Geometry: final body of the model. Coordinates: model frame, mm. A direction names the side the tool comes from. Give positions to 0.01 mm unless a question says otherwise; leave off trailing zeros. Write each loop counter-clockwise with the first axis right and the second up, starting at its lowest first coordinate (ties: lowest second). Pieces come first, ordered by that corner, then holes. Notation, with made-up numbers: M 74.25,-19 L 90.25,-19 A12 cw 90.25,-10 Z; hole C 31,58.25 d9. An arc over 180 degrees is marked long. One line per question, with ' | ' between items.
from build123d import *

# Parameters (mm, degrees)
SKETCH1_W           = 40
SKETCH1_H           = 20
BOSS_EXTRUDE1_DEPTH = 37
BOSS_EXTRUDE2_DEPTH = 2
SKETCH3_W           = 3
SKETCH3_H           = 20
BOSS_EXTRUDE3_DEPTH = 7
SKETCH4_W           = 3
SKETCH4_H           = 20
BOSS_EXTRUDE4_DEPTH = 7
SKETCH8_R           = 2.15
CUT_EXTRUDE9_DEPTH  = 7
CUT_EXTRUDE10_REACH = 44.308
SKETCH9_R           = 2.15
CUT_EXTRUDE11_REACH = 44.308
SKETCH10_R          = 2.15
SKETCH11_R          = 3
BOSS_EXTRUDE5_DEPTH = 6


with BuildPart() as part:
    # Sketch1 → Boss-Extrude1 (new body)
    with BuildSketch(Plane.XY):
        Rectangle(SKETCH1_W, SKETCH1_H)
    extrude(amount=BOSS_EXTRUDE1_DEPTH)

    # Sketch2 → Boss-Extrude2 (add)
    with BuildSketch(Plane.XY.offset(37)):
        with BuildLine():
            Line((15, 10), (15, -10))
            Line((15, -10), (-10, -10))
            ThreePointArc((-10, -10), (-20, 0), (-10, 10))
            Line((-10, 10), (15, 10))
        make_face()
    extrude(amount=BOSS_EXTRUDE2_DEPTH)

    # Sketch3 → Boss-Extrude3 (add)
    with BuildSketch(Plane(origin=(20, 0, 0), x_dir=(0, 0, -1), z_dir=(1, 0, 0))):
        with Locations((-29.5, 0)):
            Rectangle(SKETCH3_W, SKETCH3_H)
    extrude(amount=BOSS_EXTRUDE3_DEPTH)

    # Sketch4 → Boss-Extrude4 (add)
    with BuildSketch(Plane.ZY.offset(20)):
        with Locations((29.5, 0)):
            Rectangle(SKETCH4_W, SKETCH4_H)
    extrude(amount=BOSS_EXTRUDE4_DEPTH)

    # Sketch8 → Cut-Extrude9 (cut)
    with BuildSketch(Plane.XY.offset(31)):
        with Locations((-25, 6)):
            Circle(SKETCH8_R)
    extrude(amount=-CUT_EXTRUDE9_DEPTH, mode=Mode.SUBTRACT)

    # Sketch9 → Cut-Extrude10 (cut, up to next)
    with BuildSketch(Plane.XY.offset(31), mode=Mode.PRIVATE) as cut_extrude10_sk1:
        with Locations((-25, -6)):
            Circle(SKETCH9_R)
    cut_extrude10_tool1 = extrude(cut_extrude10_sk1.sketch, amount=-CUT_EXTRUDE10_REACH, mode=Mode.PRIVATE) & part.part
    add(cut_extrude10_tool1.solids().sort_by_distance((-25, -6, 31))[0], mode=Mode.SUBTRACT)

    # Sketch10 → Cut-Extrude11 (cut, up to next)
    with BuildSketch(Plane.XY.offset(31), mode=Mode.PRIVATE) as cut_extrude11_sk1:
        with Locations((25, 6)):
            Circle(SKETCH10_R)
    cut_extrude11_tool1 = extrude(cut_extrude11_sk1.sketch, amount=-CUT_EXTRUDE11_REACH, mode=Mode.PRIVATE) & part.part
    # Sketch10 → Cut-Extrude11 (cut, up to next)
    with BuildSketch(Plane.XY.offset(31), mode=Mode.PRIVATE) as cut_extrude11_sk2:
        with Locations((25, -6)):
            Circle(SKETCH10_R)
    cut_extrude11_tool2 = extrude(cut_extrude11_sk2.sketch, amount=-CUT_EXTRUDE11_REACH, mode=Mode.PRIVATE) & part.part
    add(cut_extrude11_tool1.solids().sort_by_distance((25, 6, 31))[0], mode=Mode.SUBTRACT)
    add(cut_extrude11_tool2.solids().sort_by_distance((25, -6, 31))[0], mode=Mode.SUBTRACT)

    # Sketch11 → Boss-Extrude5 (add)
    with BuildSketch(Plane.XY.offset(39)):
        with Locations((-10, 0)):
            Circle(SKETCH11_R)
    extrude(amount=BOSS_EXTRUDE5_DEPTH)


solid = part.part
(1) Set-up query: faces 5 (the face through (20, 0, 34)), 6 (the face through (23, 0, 28)), 7 (the face through (-23, 0, 31)). Return all of +Z, -Z, +X, -X, +Y, -Y with unobstructed straight access to the full face (end or side cutting, diameter ignored); none if empty.
Working result:
face 5: +Z, +X, +Y, -Y | face 6: -Z, +X, +Y, -Y | face 7: +Z, -X, +Y, -Y
(2) Draft query along X for faces 1 (the face through (-27, 8, 29)), 2 (the face through (22.85, 6.08, 29.52)), 3 (the face through (-18, -8, 37)), 4 (the face through (-22.85, 5.92, 29.52)). Return one class per face: released by +X, released by -X, zero draft, split by the parting line, or undercut.
Working result:
face 1: released by -X | face 2: undercut | face 3: zero draft | face 4: undercut
(3) First-contact query: P1, Ø3.5, axis at x = 25, y = -6, coming from the -Z side; P2, Ø4, axis at y = -2.5, z = 34.5, coming from the -X side; P3, Ø10, axis at x = -17.5, y = 3, coming from the +Z side; P4, Ø7.5, axis at x = -23.5, y = 3.5, coming from the -Z side. Flat tips, straight axial feed; report the tip coordinate or a pass-through.
Working result:
P1: passes through | P2: stops at x = -20 | P3: stops at z = 39 | P4: stops at z = 0
(4) Cut plane A-A, the plane x = -25. Return loops of the section in (y, z).
Working result:
outline: M -10,28 L -8.15,28 L -8.15,31 L -10,31 Z; M -3.85,28 L 3.85,28 L 3.85,31 L -3.85,31 Z; M 8.15,28 L 10,28 L 10,31 L 8.15,31 Z
(5) Cut plane C-C, the plane x = 10. Return loops of the section in (y, z).
Working result:
outline: M -10,0 L 10,0 L 10,39 L -10,39 Z
(6) Cut plane B-B, the plane y = 6. Return loops of the section in (x, z).
Working result:
outline: M -22.85,28 L -20,28 L -20,0 L 20,0 L 20,28 L 22.85,28 L 22.85,31 L 20,31 L 20,37 L 15,37 L 15,39 L -18,39 L -18,37 L -20,37 L -20,31 L -22.85,31 Z
(7) Cut plane D-D, the plane z = 12. Return loops of the section in (x, y), then the cut area to 3 significant figures.
Working result:
outline: M -20,-10 L 20,-10 L 20,10 L -20,10 Z | area: 800 mm^2
(8) Material intervals for L1, parallel to Y at x = -25, z = 29.95; L2, parallel to Z at x = -17.5, y = -0.25; L3, parallel to X at y = -3, z = 31.5, sorted ascending. Write a range as [from, to].
Working result:
L1: y = [-10, -8.15], [-3.85, 3.85], [8.15, 10] | L2: z = [0, 39] | L3: x = [-20, 20]
